Input: dimensioned drawing with shaded views. Units: mm. Origin: part minimum x, y, z. Give positions to 0.01 mm unless a question says otherwise; leave off trailing zeros. Loops run counter-clockwise (first coordinate to the right, second up) from the corner with the lowest first, then second, coordinate; pieces in that order, holes last. Notation, with made-up numbers: (51.5, 67) -> (73.5, 67) arc R18 cw to (73.5, 92) -> close; hole circle Ø6 at (13, -30). An arc over 180 degrees is marked (long way). One line per question, with ' | ' between items. Start each with the question number.
Item 1: Pin query (flat end, axial travel): P1, Ø4, axis at x = 11.5, y = 79.5, coming from the -Z side; P2, Ø15, axis at x = 15, y = 34, coming from the +Z side; P3, Ø0.6, axis at x = 1, z = 5, coming from the +Y side; P4, Ø0.6, axis at x = 17, y = 107.5, coming from the +Z side. Return the tip coordinate at first contact, or that it passes through.
Item 2: Material intervals for line 1 along X through (y, z) = (21, 6.25); line 2 along Y through (x, z) = (11.5, 1); line 3 along X through (y, z) = (33, 1), sorted ascending. Write a range as [from, to].
Item 3: Mould query, pull axis X, two halves, no side actions, for the marked faces 1 and 2. Classes: released by +X, released by -X, zero draft, split by the parting line, or undercut.
Item 4: Section C-C on z = 1. Return loops of the section in (x, y), then the cut area to 3 significant figures.
Item 5: Section A-A on x = 42.5. Return loops of the section in (y, z).
Item 6: Section D-D on x = 26.85. Return loops of the section in (y, z).
Item 7: Section B-B on y = 45.5. Return loops of the section in (x, z).
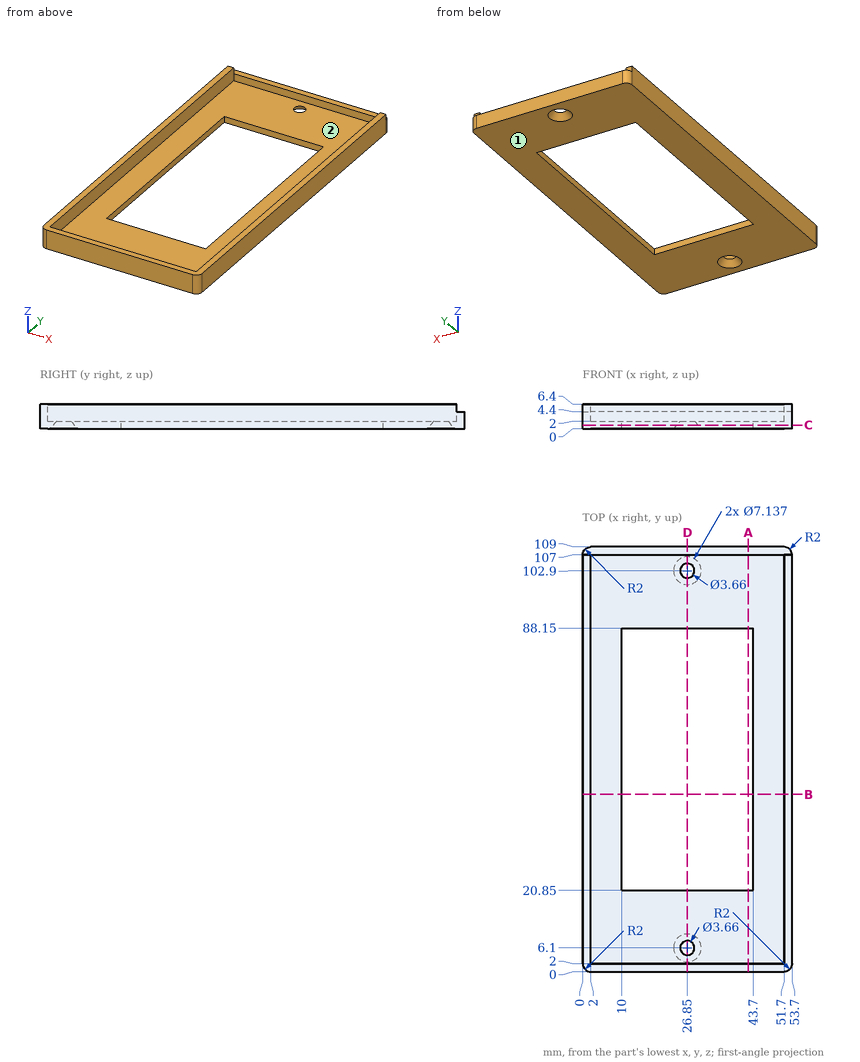
Result sheet:
1) P1: stops at z = 0 | P2: stops at z = 2 | P3: stops at y = 107 | P4: stops at z = 4.4
2) line 1: x = [0, 2], [51.7, 53.7] | line 2: y = [0, 20.85], [88.15, 109] | line 3: x = [0, 10], [43.7, 53.7]
3) face 1: zero draft | face 2: undercut
4) outline: (0, 2) arc R2 ccw to (2, 0) -> (51.7, 0) arc R2 ccw to (53.7, 2) -> (53.7, 107) arc R2 ccw to (51.7, 109) -> (2, 109) arc R2 ccw to (0, 107) -> close; hole (10, 20.85) -> (43.7, 20.85) -> (43.7, 88.15) -> (10, 88.15) -> close; hole circle Ø5.4 at (26.85, 6.1); hole circle Ø5.4 at (26.85, 102.9) | area: 3,540 mm²
5) outline: (0, 0) -> (20.85, 0) -> (20.85, 2) -> (2, 2) -> (2, 6.4) -> (0, 6.4) -> close; (88.15, 0) -> (109, 0) -> (109, 4.4) -> (107, 4.4) -> (107, 2) -> (88.15, 2) -> close
6) outline: (0, 0) -> (2.53, 0) -> (4.27, 2) -> (2, 2) -> (2, 6.4) -> (0, 6.4) -> close; (7.93, 2) -> (9.67, 0) -> (20.85, 0) -> (20.85, 2) -> close; (88.15, 0) -> (99.33, 0) -> (101.07, 2) -> (88.15, 2) -> close; (104.73, 2) -> (106.47, 0) -> (109, 0) -> (109, 4.4) -> (107, 4.4) -> (107, 2) -> close
7) outline: (0, 0) -> (10, 0) -> (10, 2) -> (2, 2) -> (2, 6.4) -> (0, 6.4) -> close; (43.7, 0) -> (53.7, 0) -> (53.7, 6.4) -> (51.7, 6.4) -> (51.7, 2) -> (43.7, 2) -> close
